Source: CAD feature listing. Evaluate the final solid. Frame: model axes, mm. A direction names the side the tool comes from. Round coordinates to 2 decimals unless told otherwise and drop trailing zeros. Write each loop counter-clockwise with the first axis right and the second up, starting at its lowest first coordinate (ties: lowest second). Pieces come first, ordered by that corner, then holes. Notation, with made-up numbers: (3, -4) -> (10, -4) arc R10 cw to (10, 11) -> close; hole circle Ø10 at (76, 24.5). An arc over 180 degrees is marked (long way). Put each result on its own line as item: value.
Solid Edge part; units mm, degrees
sketch "Sketch1" plane through (0, 0, 0) normal (0, 0, 1) x (1, 0, 0)
  circle A0 centre (0, 0) radius 3
extrude "Protrusion1" add sketch "Sketch1" along normal mid plane 6
chamfer "Chamfer1" distance 0.45 angle 45 2 edges at (-3, 0, -3) (-3, 0, 3)
sketch "Sketch2" plane through (0, 0, 3) normal (0, 0, 1) x (1, 0, 0)
  line L0 (-0.866, 1.5) -> (0.866, 1.5)
  line L1 (1.7321, 0) -> (0.866, 1.5)
  line L2 (0.866, -1.5) -> (1.7321, 0)
  line L3 (-0.866, -1.5) -> (0.866, -1.5)
  line L4 (-1.7321, 0) -> (-0.866, -1.5)
  line L5 (-0.866, 1.5) -> (-1.7321, 0)
extrude "Cutout1" cut sketch "Sketch2" against normal blind 3
properties part number "24104557"
Q1. Pin query (flat end, axial travel): pin 1 (0.9 mm diameter, centred on x = 0, y = 0, fed in from +Z). Return the tip coordinate at first contact, or that it passes through.
Ans:
pin 1: stops at z = 0
Q2. Cut plane B-B on x = 0. Output: boundary loops of the cut face in (y, z), and give its area (3 significant figures).
Ans:
outline: (-3, -2.55) -> (-2.55, -3) -> (2.55, -3) -> (3, -2.55) -> (3, 2.55) -> (2.55, 3) -> (1.5, 3) -> (1.5, 0) -> (-1.5, 0) -> (-1.5, 3) -> (-2.55, 3) -> (-3, 2.55) -> close
area: 26.6 mm^2
Q3. Material intervals for line 1 (X direction, y = 2.45, z = -2.2); line 2 (Y direction, x = -0.6, z = 2.4); line 3 (Y direction, x = -0.2, z = 1.15), sorted ascending. Write a range as [from, to].
Ans:
line 1: x = [-1.73, 1.73]
line 2: y = [-2.94, -1.5], [1.5, 2.94]
line 3: y = [-2.99, -1.5], [1.5, 2.99]
Q4. Cut plane A-A on z = 2.25. Output: boundary loops of the cut face in (x, y), and give its area (3 significant figures).
Ans:
outline: circle Ø6 at (0, 0); hole (-1.73, 0) -> (-0.87, -1.5) -> (0.87, -1.5) -> (1.73, 0) -> (0.87, 1.5) -> (-0.87, 1.5) -> close
area: 20.5 mm^2
Q5. Cut plane C-C on z = -0.1. Output: boundary loops of the cut face in (x, y), and give its area (3 significant figures).
Ans:
outline: circle Ø6 at (0, 0)
area: 28.3 mm^2
Q6. Draft query along Y for faces 1 (the cylindrical face through (-3, 0, 0)), 2 (the flat face through (0, -2, 3)), 3 (the flat face through (0, 1.5, 2)). Return one class per face: +Y half, -Y half, draft (parallel to the pull), parting line (faces both ways), or undercut.
Ans:
face 1: parting line
face 2: draft
face 3: undercut
Q7. Reachability of faces 4 (the flat face through (-1.293, 0.76, 1.521)), 5 (the flat face through (0, 0, -3)) from +Z, -Z, +X, -X, +Y, -Y: full face, straight path, thin tool, end or side. Return the list, or none.
Ans:
face 4: +Z
face 5: -Z, +X, -X, +Y, -Y
